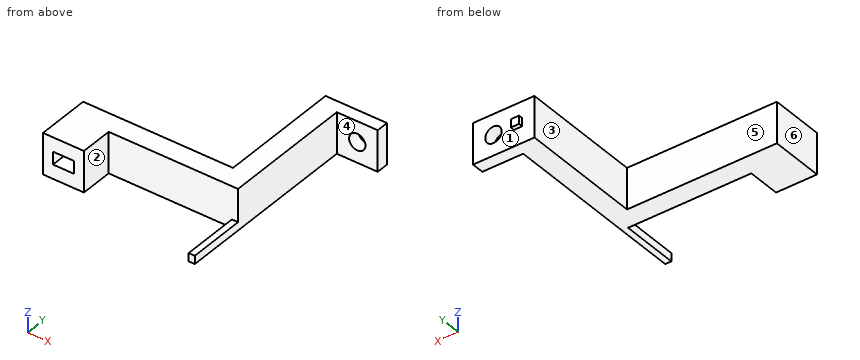
```python
from build123d import *

# Parameters (mm, degrees)
BOSS_EXTRUDE1_DEPTH = 10
SKETCH2_W           = 5.1
SKETCH2_H           = 3.1
CUT_EXTRUDE1_DEPTH  = 10
SKETCH3_W           = 2
SKETCH3_H           = 2
BOSS_EXTRUDE2_DEPTH = 1
CUT_EXTRUDE4_REACH  = 69.908
SKETCH11_R          = 2
SKETCH12_W          = 1.5
SKETCH12_H          = 2
BOSS_EXTRUDE4_DEPTH = 14


with BuildPart() as part:
    # Sketch1 → Boss-Extrude1 (new body)
    with BuildSketch(Plane.XY):
        Polygon((10, 13), (36.6, 13), (36.6, 43), (51.6, 43), (51.6, 40), (41.6, 40), (41.6, 8), (10, 8), (10, 0), (0, 0), (0, 13), align=None)
    extrude(amount=BOSS_EXTRUDE1_DEPTH)

    # Sketch2 → Cut-Extrude1 (cut)
    with BuildSketch(Plane.XZ):
        with Locations((5, 5)):
            Rectangle(SKETCH2_W, SKETCH2_H)
    extrude(amount=-CUT_EXTRUDE1_DEPTH, mode=Mode.SUBTRACT)

    # Sketch3 → Boss-Extrude2 (add)
    with BuildSketch(Plane(origin=(0, 43, 0), x_dir=(1, 0, 0), z_dir=(0, 1, 0))):
        with Locations((40.6, -5)):
            Rectangle(SKETCH3_W, SKETCH3_H)
    extrude(amount=BOSS_EXTRUDE2_DEPTH)

    # Sketch11 → Cut-Extrude4 (cut, up to next)
    with BuildSketch(Plane(origin=(0, 43, 0), x_dir=(1, 0, 0), z_dir=(0, 1, 0)), mode=Mode.PRIVATE) as cut_extrude4_sk1:
        with Locations(Location((46.6, -5, 0), (0, 0, 270))):
            Circle(SKETCH11_R)
    cut_extrude4_tool1 = extrude(cut_extrude4_sk1.sketch, amount=-CUT_EXTRUDE4_REACH, mode=Mode.PRIVATE) & part.part
    add(cut_extrude4_tool1.solids().sort_by_distance((46.6, 43, 5))[0], mode=Mode.SUBTRACT)

    # Sketch12 → Boss-Extrude4 (add)
    with BuildSketch(Plane.XZ.offset(-8)):
        with Locations((40.85, 1)):
            Rectangle(SKETCH12_W, SKETCH12_H)
    extrude(amount=BOSS_EXTRUDE4_DEPTH)


solid = part.part
```
Input: part model. Units: mm. Frame: model coordinates. Face numbers are marked on the shaded views. A direction names the side the tool comes from. Coordinates: 2 decimals unless noted, no trailing zeros. Loops run counter-clockwise (first coordinate to the right, second up) from the corner with the lowest first, then second, coordinate; pieces in that order, holes last. Notation, with made-up numbers: M 19.25,55 L 36.25,55 A21 cw 36.25,69 Z; hole C -3.75,-10 d1. An arc over 180 degrees is marked long. Use a Markdown table: item, result. Add a question column.
1) Draft query along X for the marked faces 1, 2 and 3. Return one class per face: +X half, -X half, draft (parallel to the pull), parting line (faces both ways), or undercut.
2) Section A-A, the plane z = 5. Return the cut outline in (x, y).
3) Set-up query: the marked faces 4, 5 and 6. Return all of +Z, -Z, +X, -X, +Y, -Y with unobstructed straight access to the full face (end or side cutting, diameter ignored); none if empty.
4) Section B-B, the plane x = 4. Return the cut outline in (y, z).
5) Line query: L1, parallel to X at y = 41.9, z = 5; L2, parallel to X at y = 6, z = 4; L3, parallel to Y at x = 8, z = 3.75. Output: solid intervals per line, ascending. Write a range as from..to.
6) Section C-C, the plane x = 46.6. Return the cut outline in (y, z), plus the area to 3 significant figures.
7) Pin query (flat end, axial travel): P1, Ø3, axis at y = 22.5, z = 5, coming from the +X side; P2, Ø1.5, axis at y = 6, z = 2.5, coming from the -X side; P3, Ø0.5, axis at x = 40, y = 43.5, coming from the -Z side; P4, Ø0.5, axis at x = 40, y = 43.5, coming from the +Z side. Return the tip coordinate at first contact, or that it passes through.
8) Section D-D, the plane z = 1.25. Return the cut outline in (x, y), plus the area to 3 significant figures.
Answer below:
| question | item | result |
|---|---|---|
| 1 | face 1 | draft |
| 1 | face 2 | undercut |
| 1 | face 3 | -X half |
| 2 | outline | M 0,0 L 2.45,0 L 2.45,10 L 7.55,10 L 7.55,0 L 10,0 L 10,8 L 41.6,8 L 41.6,40 L 44.6,40 L 44.6,43 L 41.6,43 L 41.6,44 L 39.6,44 L 39.6,43 L 36.6,43 L 36.6,13 L 0,13 Z; M 48.6,40 L 51.6,40 L 51.6,43 L 48.6,43 Z |
| 3 | face 4 | +Z, -Z, +X, -Y |
| 3 | face 5 | +Z, -Z, -X, +Y |
| 3 | face 6 | +Z, -Z, -X, +Y, -Y |
| 4 | outline | M 0,0 L 13,0 L 13,10 L 0,10 L 0,6.55 L 10,6.55 L 10,3.45 L 0,3.45 Z |
| 5 | L1 | 36.6..44.6, 48.6..51.6 |
| 5 | L2 | 0..2.45, 7.55..10 |
| 5 | L3 | 0..13 |
| 6 | outline | M 40,0 L 43,0 L 43,3 L 40,3 Z; M 40,7 L 43,7 L 43,10 L 40,10 Z |
| 6 | area | 18.0 mm2 |
| 7 | P1 | x = 41.6 |
| 7 | P2 | x = 0 |
| 7 | P3 | z = 4 |
| 7 | P4 | z = 6 |
| 8 | outline | M 0,0 L 10,0 L 10,8 L 40.1,8 L 40.1,-6 L 41.6,-6 L 41.6,40 L 51.6,40 L 51.6,43 L 36.6,43 L 36.6,13 L 0,13 Z |
| 8 | area | 489 mm2 |
